Can you work these out from the model? Positions are in its coordinate system, mm. Give positions to 0.01 mm unless a question says otherwise; leave off trailing zeros. Loops run counter-clockwise (first coordinate to the right, second up) from the corner with the lowest first, then second, coordinate; pieces in that order, holes last. Notation, with made-up numbers: M 72.5,53 L 77.5,53 A23 ccw 77.5,72 Z; hole C 14,-9 d5. An arc over 180 degrees is marked long. One line per item, written item: value. Start each with the question number.
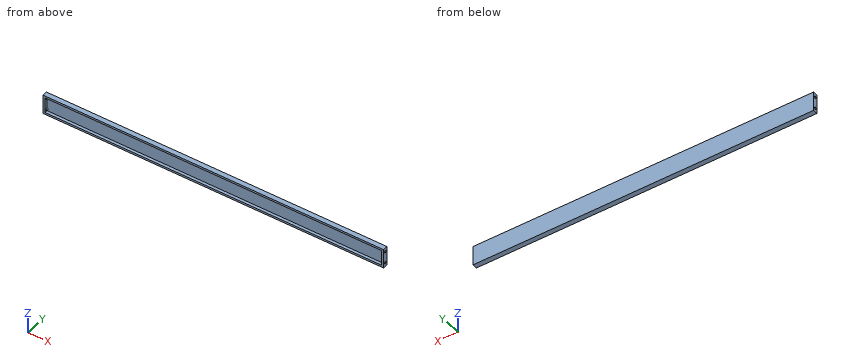
Autodesk Inventor part; units mm, degrees
ref_plane "YZ Plane" through (0, 0, 0) normal (1, 0, 0) x (0, 1, 0)
ref_plane "XZ Plane" through (0, 0, 0) normal (0, 1, 0) x (-1, 0, 0)
ref_plane "XY Plane" through (0, 0, 0) normal (0, 0, 1) x (1, 0, 0)
sketch "スケッチ1" plane through (0, 0, 0) normal (0, 0, 1) x (1, 0, 0)
  line L0 (0, 0) -> (352, 0)
  line L1 (352, 0) -> (352, 5)
  line L2 (352, 5) -> (0, 5)
  line L3 (0, 5) -> (0, 0)
  line L4 (0, 0) -> (6, 0)
  line L5 (0, 1) -> (0, 0)
  dimension "d0" = 352
  dimension "d1" = 5
extrude "押し出し1" add sketch "スケッチ1" along normal blind 20
sketch "スケッチ3" plane through (0, 0, 0) normal (-1, 0, 0) x (0, 0, 1)
  line L0 (0, 5) -> (0, 0)
  line L1 (0, 0) -> (20, 0)
  line L2 (20, 5) -> (20, 0)
  line L3 (0, 5) -> (20, 5)
  circle A0 centre (4, 2.5) radius 1.2
  circle A1 centre (16, 2.5) radius 1.2
  dimension "d14" = 2.4
  dimension "d15" = 2.4
  dimension "d16" = 2.5
  dimension "d17" = 4
  dimension "d18" = 4
  dimension "d19" = 2.5
extrude "押し出し3" cut sketch "スケッチ3" against normal blind 3 contours A0 | A1
sketch "スケッチ4" plane through (0, 0, 0) normal (0, -1, 0) x (1, 0, 0)
  line L0 (0, 0) -> (352, 0)
  line L1 (352, 0) -> (352, 20)
  line L2 (0, 20) -> (352, 20)
  line L3 (0, 0) -> (0, 20)
  line L4 (2, 2) -> (350, 2)
  line L5 (350, 2) -> (350, 18)
  line L6 (350, 18) -> (2, 18)
  line L7 (2, 18) -> (2, 2)
  dimension "d22" = 2
  dimension "d23" = 2
  dimension "d24" = 2
  dimension "d25" = 2
extrude "押し出し4" cut sketch "スケッチ4" against normal blind 3 contours L7 L6 L5 L4
sketch "スケッチ5" plane through (352, 0, 0) normal (1, 0, 0) x (0, 0, -1)
  arc A0 (-5.0909, 3) -> (-2.9091, 3) centre (-4, 2.5) ccw
  arc A1 (-2.9091, 3) -> (-5.0909, 3) centre (-4, 2.5) ccw
  arc A2 (-17.0909, 3) -> (-14.9091, 3) centre (-16, 2.5) ccw
  arc A3 (-14.9091, 3) -> (-17.0909, 3) centre (-16, 2.5) ccw
extrude "押し出し5" cut sketch "スケッチ5" against normal blind 3
properties part number "arm1_L" material "アルミニウム 6061"
Q1. I need wall thicknesses on line 1 along Z through (x, y) = (350.65, 2.5); line 2 along X through (y, z) = (0.6, 4.5); line 3 along Y through (x, z) = (350.55, 16). Which ranges of each line are inside material? Lowest first, please.
Q2. For P1, Ø12, axis at x = 157, z = 15, coming from the -Y side; P2, Ø1.9, axis at y = 2.5, z = 4, coming from the -X side; P3, Ø2, axis at y = 2.5, z = 4, coming from the +X side; P4, Ø8, axis at x = 63.5, z = 12, coming from the -Y side, each with a flat end and sliding along its axis, tell me the tip position at first contact or that it passes through.
Q3. If we section it at A-A, the plane x = 321: Write out the boundary of the cut face in (y, z), plus the area to 3 significant figures.
Response:
1. line 1: 0 to 2.8, 5.2 to 14.8, 17.2 to 20
1. line 2: 0 to 2, 350 to 352
1. line 3: 0 to 1.3, 3.7 to 5
2. P1: y = 0
2. P2: x = 3
2. P3: x = 349
2. P4: y = 3
3. outline: M 0,0 L 5,0 L 5,20 L 0,20 L 0,18 L 3,18 L 3,2 L 0,2 Z
3. area: 52.0 mm^2
